Design review of the part built by this model. Coordinates are the model's own, in mm. Face numbers are marked on the shaded views. Coordinates: 2 decimals unless noted, no trailing zeros. Write each loop counter-clockwise with the first axis right and the second up, starting at its lowest first coordinate (ties: lowest second). Pieces come first, ordered by that corner, then holes. Notation, with made-up numbers: (76, -16.75) -> (97, -16.75) arc R20 ccw to (97, -7.75) -> close; hole circle Ø5 at (24.5, -19.75). An arc over 180 degrees is marked (long way). Return JSON: item names as keys, results as strings. Group by question number.
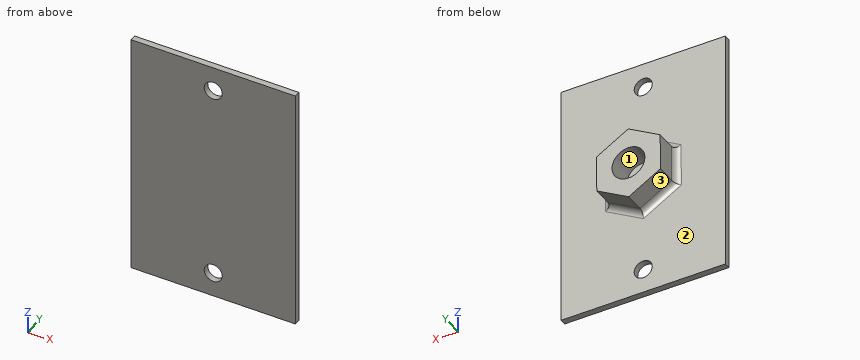
from build123d import *

# Parameters (mm, degrees)
SKETCH1_R      = 2
EXTRUDE1_DEPTH = 3.125
SKETCH2_R      = 1.1
EXTRUDE2_DEPTH = 0.75
FILLET1_R      = 0.75


with BuildPart() as part:
    # Sketch1 → Extrude1 (new body)
    with BuildSketch(Plane(origin=(0, 0, 0), x_dir=(1, 0, 0), z_dir=(0, 1, 0))):
        Polygon((3.859462612, 2.263930582), (-0.030890091, 4.474357958), (-3.890352703, 2.210427376), (-3.859462612, -2.263930582), (0.030890091, -4.474357958), (3.890352703, -2.210427376), align=None)
        with Locations(Location((0, 0, 0), (0, 0, 270))):  # turned: the seam where the file's is
            Circle(SKETCH1_R, mode=Mode.SUBTRACT)
    extrude(amount=EXTRUDE1_DEPTH)

    # Sketch2 → Extrude2 (add)
    with BuildSketch(Plane.XZ):
        Polygon((10, 0), (10, -15), (-10, -15), (-10, 15), (10, 15), align=None)
        with Locations(Location((0, -12, 0), (0, 0, 270))):  # turned: the seam where the file's is
            Circle(SKETCH2_R, mode=Mode.SUBTRACT)
        with Locations(Location((0, 12, 0), (0, 0, 90))):  # turned: the seam where the file's is
            Circle(SKETCH2_R, mode=Mode.SUBTRACT)
    extrude(amount=EXTRUDE2_DEPTH)

    # Fillet1
    fillet1_edges = [part.edges().sort_by_distance(p)[0] for p in [
        (1.960621397, 0, 3.342392667),
        (-1.91428626, 0, 3.36914427),
        (-3.874907657, 0, 0.026751603),
        (-1.960621397, 0, -3.342392667),
        (1.91428626, 0, -3.36914427),
        (3.874907657, 0, -0.026751603),
    ]]
    fillet(fillet1_edges, radius=FILLET1_R)


solid = part.part
Q1. For P1, Ø1.5, axis at x = 4.5, z = -4.5, coming from the +Y side; P2, Ø2, axis at x = 1, z = 0.5, coming from the +Y side (3 decimals); P3, Ø1.5, axis at y = 1.5, z = 0, coming from the +X side, all flat-tipped, find the tip position at first contact; note any pin that passes through.
Q2. We need section A-A on z = 12. Write out the cut boundary in (x, y).
Q3. We need section C-C on x = -5.25. Write out the cut boundary in (y, z), plus the area to 3 significant figures.
Q4. The part is to be moulded in two halves that separate along X. For the marked faces 1, 2 and 3, say which applies: +X half, -X half, draft (parallel to the pull), parting line (faces both ways), or undercut.
Q5. Wall thickness on L1, parallel to X at y = -0.2, z = 12; L2, parallel to Y at x = -4.5, z = 10.5; L3, parallel to X at y = 1.85, z = 0: over which ranges is each line inside the solid? List them lowest first.
Q6. We need section D-D on z = -6.75. Write out the cut boundary in (x, y).
Q7. We need section B-B on y = 1.3. Write out the cut boundary in (x, z), plus the area to 3 significant figures.
Findings below:
{
 "1": {"P1": "stops at y = 0", "P2": "stops at y = 3.125", "P3": "stops at x = 3.88"},
 "2": {"outline": "(-10, -0.75) -> (-1.1, -0.75) -> (-1.1, 0) -> (-10, 0) -> close; (1.1, -0.75) -> (10, -0.75) -> (10, 0) -> (1.1, 0) -> close"},
 "3": {"outline": "(-0.75, -15) -> (0, -15) -> (0, 15) -> (-0.75, 15) -> close", "area": "22.5 mm^2"},
 "4": {"face 1": "undercut", "face 2": "draft", "face 3": "-X half"},
 "5": {"L1": "x = -10 to -1.1, 1.1 to 10", "L2": "y = -0.75 to 0", "L3": "x = -3.88 to -2, 2 to 3.88"},
 "6": {"outline": "(-10, -0.75) -> (10, -0.75) -> (10, 0) -> (-10, 0) -> close"},
 "7": {"outline": "(-3.89, -2.21) -> (-0.03, -4.47) -> (3.86, -2.26) -> (3.89, 2.21) -> (0.03, 4.47) -> (-3.86, 2.26) -> close; hole circle Ø4 at (0, 0)", "area": "39.4 mm^2"}
}
